```python
from build123d import *

# Parameters (mm, degrees)
F1_W     = 19.101374
F1_H     = 59.278082
F3_W     = 29.123306
F3_H     = 27.092062
F4_DEPTH = 76.2
F5_R     = 12.7
F6_DEPTH = 12.7


with BuildPart() as f2:
    # F1 (on Front) → F2 (revolve)
    with BuildSketch(Plane.XZ):
        with Locations((-43.324234, 6.909995)):
            Rectangle(F1_W, F1_H)
    revolve(axis=Axis((0, 0, -2.969272), (0, 0, -1)))

    # F3 (on face) → F4 (cut)
    with BuildSketch(Plane.XY.offset(36.549036)):
        with Locations((27.437061, 0.549149)):
            Rectangle(F3_W, F3_H)
    extrude(amount=-F4_DEPTH, mode=Mode.SUBTRACT)

    # F5 (on Front) → F6 (cut, symmetric)
    with BuildSketch(Plane.XZ):
        Circle(F5_R)
    extrude(amount=F6_DEPTH, both=True, mode=Mode.SUBTRACT)


solid = f2.part
```
Geometry check sheet. Reference: the model listing, model coordinates, mm. A direction names the side the tool comes from. Coordinates: 2 decimals unless noted, no trailing zeros. Write each loop counter-clockwise with the first axis right and the second up, starting at its lowest first coordinate (ties: lowest second). Pieces come first, ordered by that corner, then holes. Notation, with made-up numbers: M -34,-39 L -2,-39 A22 ccw -2,-13 Z; hole C -2,-31.75 d3. An arc over 180 degrees is marked long. One line per item, written item: value. Start each with the question number.
(1) Depth check by flat-ended pin: pin 1 (1 mm diameter, centred on y = 14.5, z = 14.5, fed in from -X); pin 2 (12 mm diameter, centred on x = 34, z = -3.5, fed in from +Y); pin 3 (1.5 mm diameter, centred on y = -15, z = 29.5, fed in from -X); pin 4 (8 mm diameter, centred on x = 11, y = -26.5, fed in from +Z). Enter the tip coordinate at first touch or a pass-through.
(2) Sectioned sample at D-D, the plane y = -44. Enter the section's corners in (x, z).
(3) Tool access check on faces 1 (the face through (41.999, 0, 7)), 2 (the face through (-35, 1, -22.729)). Record the directions out of +Z, -Z, +X, -X, +Y, -Y that give a thin tool (end or side, any length) a straight path to the whole face; none if there is none.
(4) Scan lines: line 1 along X through (y, z) = (-1, 29); line 2 along Y through (x, z) = (0, 15); line 3 along Y through (x, z) = (4.5, 9). Record each from-to range of solid material in increasing order. Write a range as [from, to].
(5) Sectioned sample at A-A, the plane x = 0. Enter the section's corners in (y, z).
(6) Release check for a two-part mould opening along Y. For faces 3 (the face through (11.46, -51.62, 7.32)), 4 (the face through (37, -12.997, 7)), 5 (the face through (-35, 1, 36.549)) record: released by +Y, released by -Y, zero draft, split by the parting line, or undercut.
(7) Sectioned sample at C-C, the plane z = -8. Enter the section's corners in (x, y), and give its area (3 significant figures).
(8) Sectioned sample at B-B, the plane y = 0. Enter the section's corners in (x, z).
Filled sheet:
1. pin 1: x = -50.99
1. pin 2: y = 44.85
1. pin 3: x = -50.92
1. pin 4: through
2. outline: M -29.32,-22.73 L 29.32,-22.73 L 29.32,36.55 L -29.32,36.55 Z
3. face 1: +Z, -Z
3. face 2: -Z, +X, -X, +Y, -Y
4. line 1: [-52.87, -33.76], [42, 52.87]
4. line 2: [-52.87, -33.77], [33.77, 52.87]
4. line 3: [-52.68, -33.47], [33.47, 52.68]
5. outline: M -52.87,-22.73 L -33.77,-22.73 L -33.77,36.55 L -52.87,36.55 Z; M 33.77,-22.73 L 52.87,-22.73 L 52.87,36.55 L 33.77,36.55 Z
6. face 3: split by the parting line
6. face 4: undercut
6. face 5: zero draft
7. outline: C 0,0 d105.75; hole M 30.69,14.1 A33.77 ccw long 31.17,-13 L 42,-13 L 42,14.1 Z
7. area: 4,950 mm²
8. outline: M -52.87,-22.73 L -33.77,-22.73 L -33.77,36.55 L -52.87,36.55 Z; M 42,-22.73 L 52.87,-22.73 L 52.87,36.55 L 42,36.55 Z
